Autodesk Fusion 360 part; units mm, degrees
sketch "Sketch1" plane through (0, 0, 0) normal (1, 0, 0) x (0, 1, 0)
  line L0 (0, 0) -> (30, 0)
  line L1 (30, 0) -> (30, 16.161)
  line L2 (30, 16.161) -> (0, 16.161)
  line L3 (0, 16.161) -> (0, 0)
  line L4 (15, 0) -> (15, 16.161)
  dimension "d1" = 30
extrude "Extrude1" add sketch "Sketch1" along normal blind 25
sketch "Sketch2" plane through (0, 0, 0) normal (0, -1, 0) x (1, 0, 0)
  line L0 (0, 16.161) -> (0, 0)
  line L1 (0, 0) -> (25, 0)
  line L2 (25, 0) -> (25, 16.161)
  line L3 (25, 16.161) -> (0, 16.161)
  circle A0 centre (12.5, 8.0805) radius 2.35
  dimension "d4" = 4.7
sketch "Sketch3" plane through (0, 0, 0) normal (0, -1, 0) x (1, 0, 0)
sketch "Sketch4" plane through (0, 30, 0) normal (0, 1, 0) x (-1, 0, 0)
  line L0 (0, 0) -> (0, 16.161)
  line L1 (0, 16.161) -> (-25, 16.161)
  line L2 (-25, 16.161) -> (-25, 0)
  line L3 (-25, 0) -> (0, 0)
  circle A0 centre (-12.5, 8.0805) radius 2.4
  dimension "d5" = 4.8
extrude "Extrude2" cut sketch "Sketch4" against normal blind 10 contours A0
extrude "Extrude3" cut sketch "Sketch2" against normal blind 10 contours A0
sketch "Sketch5" plane through (0, 0, 0) normal (0, -1, 0) x (1, 0, 0)
  circle A0 centre (12.5, 8.0805) radius 2.35
  line L0 (0, 16.161) -> (0, 0)
  line L1 (0, 0) -> (25, 0)
  line L2 (25, 0) -> (25, 16.161)
  line L3 (25, 16.161) -> (0, 16.161)
  circle A1 centre (12.5, 8.0805) radius 7.5
  dimension "d10" = 15
extrude "Extrude4" cut sketch "Sketch5" against normal blind 45 contours L0 L1 L2 L3
Model file for the job. Use its own axes, mm. A direction names the side the tool comes from. Coordinates: 2 decimals unless noted, no trailing zeros. Order: outer loops, then holes, each group sorted by start corner. A loop starts at its lowest first (then second) coordinate and runs counter-clockwise, first axis right, second up. Notation, with made-up numbers: (-25, -38) -> (-1, -38) arc R20 ccw to (-1, -22) -> close; hole circle Ø1 at (-15.5, 81). An arc over 180 degrees is marked (long way). Return JSON: item names as keys, results as strings. Group by question number.
Item 1: Saw through at B-B on z = 7.5. Write the cut outline in (x, y).
Item 2: Saw through at A-A on x = 12.5. Write the cut outline in (y, z).
Item 3: Pull direction X, two halves, no side cores. Call faces 4 (the flat face through (12, 10, 8)), 5 (the cylindrical face through (5, 15, 8)), 6 (the flat face through (10.7, 0, 9.9)): pulls with the +X half, pulls with the -X half, needs draft (parallel to the pull), parting line crosses it, or undercut.
Item 4: Wall check: line 1 along Z through (x, y) = (12.5, 4.5); line 2 along Y through (x, z) = (11.5, 8); line 3 along Z through (x, y) = (12.5, 26). Give the ranges that are in metal, low to high. Write a range as [from, to].
Item 5: Saw through at D-D on y = 13. Write the cut outline in (x, z).
Item 6: Tool access for faces 1 (the cylindrical face through (10.6, 4.9, 6.7)), 2 (the flat face through (13, 20, 8)), 3 (the flat face through (11, 30, 6)): list every direction of +Z, -Z, +X, -X, +Y, -Y with a clear straight run to the whole face (end or side of a thin tool).
Item 7: Saw through at C-C on y = 25.25. Write the cut outline in (x, z), then the cut area to 3 significant figures.
Item 8: Flat gauge pins, fed straight in: P1, Ø3, axis at x = 12.5, z = 8.08, coming from the -Y side; P2, Ø2, axis at x = 8, z = 10, coming from the -Y side; P3, Ø1.4, axis at x = 12.5, z = 8, coming from the +Y side; P4, Ø2, axis at y = 19, z = 4.5, coming from the -X side. Where does each tip first touch, or does it go through?
Values found:
{
 "1": {"outline": "(5.02, 0) -> (10.22, 0) -> (10.22, 10) -> (14.78, 10) -> (14.78, 0) -> (19.98, 0) -> (19.98, 30) -> (14.83, 30) -> (14.83, 20) -> (10.17, 20) -> (10.17, 30) -> (5.02, 30) -> close"},
 "2": {"outline": "(0, 0.58) -> (30, 0.58) -> (30, 5.68) -> (20, 5.68) -> (20, 10.48) -> (30, 10.48) -> (30, 15.58) -> (0, 15.58) -> (0, 10.43) -> (10, 10.43) -> (10, 5.73) -> (0, 5.73) -> close"},
 "3": {"face 4": "undercut", "face 5": "parting line crosses it", "face 6": "needs draft"},
 "4": {"line 1": "z = [0.58, 5.73], [10.43, 15.58]", "line 2": "y = [10, 20]", "line 3": "z = [0.58, 5.68], [10.48, 15.58]"},
 "5": {"outline": "circle Ø15 at (12.5, 8.08)"},
 "6": {"face 1": "-Y", "face 2": "+Y", "face 3": "+Z, -Z, +X, -X, +Y"},
 "7": {"outline": "circle Ø15 at (12.5, 8.08); hole circle Ø4.8 at (12.5, 8.08)", "area": "159 mm2"},
 "8": {"P1": "stops at y = 10", "P2": "stops at y = 0", "P3": "stops at y = 20", "P4": "stops at x = 5.46"}
}
